The drawing under review shows one solid part. Ordinate dimensions are in mm from its lowest x, y, z. A direction names the side the tool comes from. Give positions to 0.01 mm unless a question says otherwise; leave off trailing zeros. Order: outer loops, then holes, each group sorted by start corner. A loop starts at its lowest first (then second) coordinate and runs counter-clockwise, first axis right, second up. Notation, with made-up numbers: (48.25, -29) -> (67.25, -29) arc R20 cw to (67.25, -1) -> close; hole circle Ø6 at (89, -33.5). An arc over 180 degrees is marked (long way). Use CSV: the item, a comma, the result in double quotes. Start each with the question number.
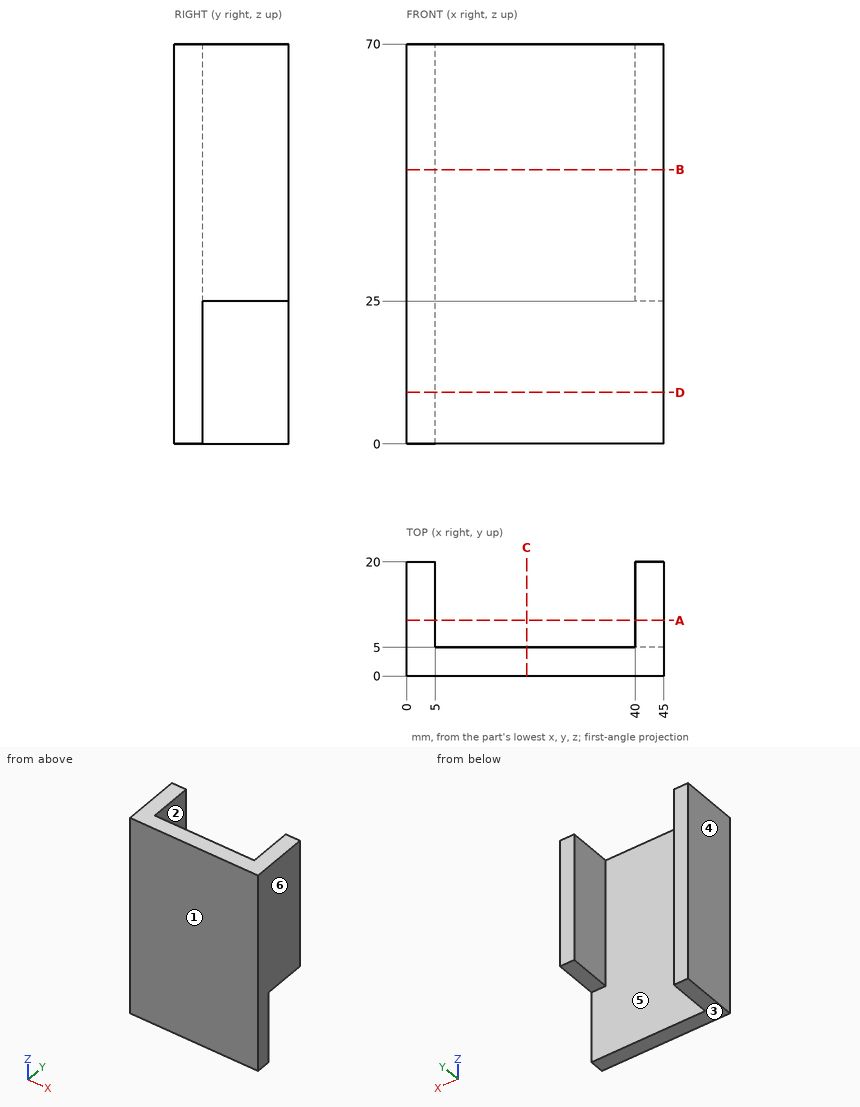
1. Consider section C-C (x = 21). State the section outline as (y, z) points, plus the area to 3 significant figures.
2. Consider section A-A (y = 9.75). State the section outline as (x, z) points, plus the area to 3 significant figures.
3. Consider section B-B (z = 48). State the section outline as (x, y) points.
4. For the marked faces 1 and 2, list the 3-axis set-ups (+Z, -Z, +X, -X, +Y, -Y) from which the entire face can be reached by the end or side of a thin tool; tool diameter is ignored.
5. Consider section D-D (z = 9). State the section outline as (x, y) points, plus the area to 3 significant figures.
6. To check wall thickness, follow L1, parallel to X at y = 14, z = 65; L2, parallel to X at y = 13.75, z = 11.5. State the ranges of each line that lie inside material, in increasing order. Write a range as [from, to].
7. Clearance check with flat-ended pins moving along their axes: P1, Ø8, axis at x = 32, y = 12.5, coming from the +Z side; P2, Ø1.5, axis at x = 43, y = 16, coming from the -Z side. State where each tip first meets the part, or that it passes through.
8. Draft analysis for pull direction X (two halves, no side actions). For the marked faces 3, 4, 5 and 6, state which applies: +X half, -X half, draft (parallel to the pull), parting line (faces both ways), or undercut.
Answer list:
1,outline,"(0, 0) -> (5, 0) -> (5, 70) -> (0, 70) -> close"
1,area,"350 mm2"
2,outline,"(0, 0) -> (5, 0) -> (5, 70) -> (0, 70) -> close; (40, 25) -> (45, 25) -> (45, 70) -> (40, 70) -> close"
2,area,"575 mm2"
3,outline,"(0, 0) -> (45, 0) -> (45, 20) -> (40, 20) -> (40, 5) -> (5, 5) -> (5, 20) -> (0, 20) -> close"
4,face 1,"+Z, -Z, +X, -X, -Y"
4,face 2,"+Z, -Z, +Y"
5,outline,"(0, 0) -> (45, 0) -> (45, 5) -> (5, 5) -> (5, 20) -> (0, 20) -> close"
5,area,"300 mm2"
6,L1,"[0, 5], [40, 45]"
6,L2,"[0, 5]"
7,P1,"through"
7,P2,"z = 25"
8,face 3,"draft"
8,face 4,"-X half"
8,face 5,"undercut"
8,face 6,"+X half"
